```python
from build123d import *

# Parameters (mm, degrees)
BOSS_EXTRUDE1_DEPTH         = 9.525
F_6_0_204_DIAMETER_HOLE1_D  = 5.1816
F_1_4_0_25_DIAMETER_HOLE1_D = 6.35


with BuildPart() as part:
    # Sketch2 → Boss-Extrude1 (new, symmetric)
    with BuildSketch(Plane.XY):
        with BuildLine():
            Line((-6.35, 0), (6.35, 0))
            Line((6.35, 0), (6.35, 12.7))
            Line((6.35, 12.7), (5.55625, 12.7))
            ThreePointArc((5.55625, 12.7), (4.994983992, 12.467516008), (4.7625, 11.90625))
            Line((4.7625, 11.90625), (4.7625, 3.1623))
            ThreePointArc((4.7625, 3.1623), (4.301251759, 2.048748241), (3.1877, 1.5875))
            Line((3.1877, 1.5875), (-5.55625, 1.5875))
            ThreePointArc((-5.55625, 1.5875), (-6.117516008, 1.355016008), (-6.35, 0.79375))
            Line((-6.35, 0.79375), (-6.35, 0))
        make_face()
    extrude(amount=BOSS_EXTRUDE1_DEPTH, both=True)

    # #6 (0.204) Diameter Hole1 (through all)
    with Locations(Plane(origin=(0, 1.5875, 0), x_dir=(1, 0, 0), z_dir=(0, 1, 0))):
        with Locations((-1.184275, 0)):
            Hole(F_6_0_204_DIAMETER_HOLE1_D / 2)

    # 1/4 (0.25) Diameter Hole1 (through all)
    with Locations(Plane.ZY.offset(-4.7625)):
        with Locations((0, 7.534275)):
            Hole(F_1_4_0_25_DIAMETER_HOLE1_D / 2)


solid = part.part
```
Geometry: final body of the model. Coordinates: model frame, mm. A direction names the side the tool comes from. Round coordinates to 2 decimals unless told otherwise and drop trailing zeros. Write each loop counter-clockwise with the first axis right and the second up, starting at its lowest first coordinate (ties: lowest second). Pieces come first, ordered by that corner, then holes.
Item 1: Pin query (flat end, axial travel): P1, Ø1.5, axis at x = 3.5, y = 2, coming from the +Z side (3 decimals); P2, Ø2.5, axis at y = 7, z = 2, coming from the -X side; P3, Ø2.5, axis at x = -2.5, z = -4, coming from the +Y side. Return the tip coordinate at first contact, or that it passes through.
Item 2: Section query D-D (z = 5.75). Return loops of the section in (x, y), plus the area to 3 significant figures.
Item 3: Section query C-C (x = -2.75). Return loops of the section in (y, z) (1 decimal).
Item 4: Section query A-A (z = 0). Return loops of the section in (x, y).
Item 5: Mould query, pull axis Z, two halves, no side actions, for faces 1 (the face through (4.762, 4.7, 2.3)), 2 (the face through (5.567, 4.435, 0.688)), 3 (the face through (3, 1, 9.525)). Classes: +Z half, -Z half, draft (parallel to the pull), parting line (faces both ways), or undercut.
Item 6: Material intervals for L1, parallel to Y at x = 5.55, z = 0; L2, parallel to X at y = 5.5, z = 6.25; L3, parallel to Y at x = -0.25, z = 7.75, sorted ascending.
Item 7: Set-up query: faces 4 (the face through (0.87, 0.78, 1.58)), 5 (the face through (1, 1.588, 2)). Return all of +Z, -Z, +X, -X, +Y, -Y with unobstructed straight access to the full face (end or side cutting, diameter ignored); none if empty.
Completed:
1. P1: stops at z = 9.525
1. P2: stops at x = 4.76
1. P3: stops at y = 1.59
2. outline: (-6.35, 0) - (6.35, 0) - (6.35, 12.7) - (5.56, 12.7) arc R0.79 ccw to (4.76, 11.91) - (4.76, 3.16) arc R1.57 cw to (3.19, 1.59) - (-5.56, 1.59) arc R0.79 ccw to (-6.35, 0.79) - close
2. area: 38.1 mm2
3. outline: (0, -9.5) - (1.6, -9.5) - (1.6, -2.1) - (0, -2.1) - close; (0, 2.1) - (1.6, 2.1) - (1.6, 9.5) - (0, 9.5) - close
4. outline: (-6.35, 0) - (-3.78, 0) - (-3.78, 1.59) - (-5.56, 1.59) arc R0.79 ccw to (-6.35, 0.79) - close; (1.41, 0) - (6.35, 0) - (6.35, 4.36) - (4.76, 4.36) - (4.76, 3.16) arc R1.57 cw to (3.19, 1.59) - (1.41, 1.59) - close; (4.76, 10.71) - (6.35, 10.71) - (6.35, 12.7) - (5.56, 12.7) arc R0.79 ccw to (4.76, 11.91) - close
5. face 1: draft
5. face 2: undercut
5. face 3: +Z half
6. L1: y = 0 to 4.36, 10.71 to 12.7
6. L2: x = 4.76 to 6.35
6. L3: y = 0 to 1.59
7. face 4: +Y, -Y
7. face 5: +Z, -Z, -X, +Y
